Check sheet for the modelled part. Datum: model origin and axes. Units: mm. A direction names the side the tool comes from. Coordinates: 2 decimals unless noted, no trailing zeros. Loops run counter-clockwise (first coordinate to the right, second up) from the corner with the lowest first, then second, coordinate; pieces in that order, holes last. Notation, with made-up numbers: M -2.75,-27 L 33.25,-27 A7 ccw 33.25,-21 Z; hole C -25,79.5 d10. An arc over 180 degrees is marked long. Answer in a Markdown table with one row per item. Add a question column.
Autodesk Inventor part; units mm, degrees
ref_plane "YZ Plane" through (0, 0, 0) normal (1, 0, 0) x (0, 1, 0)
ref_plane "XZ Plane" through (0, 0, 0) normal (0, 1, 0) x (-1, 0, 0)
ref_plane "XY Plane" through (0, 0, 0) normal (0, 0, 1) x (1, 0, 0)
sketch "Эскиз1" plane through (0, 0, 0) normal (0, 0, 1) x (1, 0, 0)
  line L0 (3, 0) -> (22.75, 0)
  line L1 (22.75, 0) -> (22.75, 13)
  line L2 (22.75, 13) -> (3, 13)
  line L3 (0, 10) -> (0, 3)
  circle A0 centre (16.25, 6.5) radius 8 construction
  circle A1 centre (16.25, 6.5) radius 2.5
  circle A2 centre (4.5, 6.5) radius 1.5
  line L4 (0, 6.5) -> (22.75, 6.5) construction
  circle A3 centre (4.5, 6.5) radius 2.75 construction
  line L5 (3, 13) -> (0, 10)
  line L6 (0, 3) -> (3, 0)
  circle A4 centre (16.25, 6.5) radius 3.75
  point P0 (0, 0)
  point P1 (0, 13)
  dimension "d0" = 16
  dimension "d3" = 3
  dimension "d6" = 5.5
  dimension "d7" = 1
  dimension "d9" = 3
  dimension "d10" = 3
  dimension "d11" = 3
  dimension "d12" = 3
  dimension "d13" = 7.5
  dimension "d23" = 6.5
  dimension "d24" = 6.5
extrude "Выдавливание1" add sketch "Эскиз1" along normal blind 3 contours L6 L3 L5 L2 L1 L0
extrude "Выдавливание2" add sketch "Эскиз1" along normal blind 14 contours A4
extrude "Выдавливание3" add sketch "Эскиз1" along normal blind 19 contours A1
chamfer "Фаска1" distance 2 angle 45 1 edges at (12.5, 6.5, 3)
properties part number "Концентратор"
Q1. Go/stop test with flat-tipped pins: pin 1 (1.5 mm diameter, centred on y = 7, z = 9.5, fed in from +X); pin 2 (1 mm diameter, centred on x = 20.5, y = 3.5, fed in from +Z); pin 3 (1 mm diameter, centred on y = 3.5, z = 11.5, fed in from +X). Record where each tip stops, or that it passes through.
Q2. Cross-section at A-A (x = 5.25). Record the cut outline in (y, z).
Q3. Access from +Z, -Z, +X, -X, +Y, -Y to the whole of each face (thin tool, end or side, straight path). Record for faces 4 (the face through (13.752, 6.39, 16.465)), 5 (the face through (0, 7, 1)).
Q4. Cross-section at B-B (x = 16.25). Record the cut outline in (y, z).
Q5. Thickness scan on L1, parallel to Y at x = 4.5, z = 1; L2, parallel to Z at x = 7.75, y = 1; L3, parallel to Z at x = 14, y = 8.5. Record the ranges inside material, lowest first.
Q6. Mould release check, pull along X, two halves, no side actions. Record for faces 1 (the face through (13.274, 8.782, 9.437)), 2 (the face through (5.886, 7.075, 1.479)), 3 (the face through (13, 0, 1)): released by +X, released by -X, zero draft, split by the parting line, or undercut.
Q7. Cross-section at C-C (z = 10.5). Record the cut outline in (x, y), plus the area to 3 significant figures.
Answer key:
| question | item | result |
|---|---|---|
| 1 | pin 1 | x = 20 |
| 1 | pin 2 | z = 4.05 |
| 1 | pin 3 | x = 19.05 |
| 2 | outline | M 0,0 L 5.2,0 L 5.2,3 L 0,3 Z; M 7.8,0 L 13,0 L 13,3 L 7.8,3 Z |
| 3 | face 4 | +Z |
| 3 | face 5 | +Z, -Z, -X, +Y, -Y |
| 4 | outline | M 0,0 L 13,0 L 13,3 L 12.25,3 L 10.25,5 L 10.25,14 L 9,14 L 9,19 L 4,19 L 4,14 L 2.75,14 L 2.75,5 L 0.75,3 L 0,3 Z |
| 5 | L1 | 0 to 5, 8 to 13 |
| 5 | L2 | 0 to 3 |
| 5 | L3 | 0 to 14 |
| 6 | face 1 | split by the parting line |
| 6 | face 2 | undercut |
| 6 | face 3 | zero draft |
| 7 | outline | C 16.25,6.5 d7.5 |
| 7 | area | 44.2 mm^2 |
